Check sheet for the modelled part. Datum: model origin and axes. Units: mm. A direction names the side the tool comes from. Give positions to 0.01 mm unless a question says otherwise; leave off trailing zeros. Write each loop counter-clockwise with the first axis right and the second up, starting at its lowest first coordinate (ties: lowest second). Pieces come first, ordered by that corner, then holes. Notation, with made-up numbers: (59.5, -4.5) -> (81.5, -4.5) arc R28 ccw to (81.5, 16.5) -> close; hole circle Ø4 at (85.25, 19). An arc over 180 degrees is marked (long way). Use a Markdown table: item, result. Add a question column.
1. Gauge pin test, flat ends, axial feed: P1, Ø10, axis at y = 31, z = 32, coming from the -X side; P2, Ø16.5, axis at x = 36, y = 30.5, coming from the -Z side; P3, Ø2.5, axis at y = 51.5, z = -15.5, coming from the -X side; P4, Ø1, axis at x = 34.5, z = 134, coming from the +Y side. Record the tip position at first contact, or that the pin passes through.
2. Set-up check for faces 1 (the flat face through (33, 45, 12)), 2 (the cylindrical face through (239.3, 2.85, 3.01)), 3 (the flat face through (148, 15, 98)), 4 (the cylindrical face through (60.7, 59.99, 2.85)), 5 (the flat face through (260, 45, 148)): record each of +Z, -Z, +X, -X, +Y, -Y from which the full face is reachable in a straight line by a thin tool's end or side.
3. Cross-section at A-A (z = 214). Enter the section's corners in (x, y).
4. Cross-section at B-B (x = 57). Enter the section's corners in (y, z), then the cut area to 3 significant figures.
5. Scan lines: probe 1 along X at (y, z) = (30.1, 167.5); probe 2 along Z at (x, y) = (175, 69); probe 3 along Y at (x, z) = (98.5, 108.5). Record each from-to range of solid material in increasing order. Write a range as [from, to].
6. Cross-section at D-D (y = 75). Enter the section's corners in (x, z), then the cut area to 3 significant figures.
7. Cross-section at C-C (z = 176). Enter the section's corners in (x, y).
8. Release check for a two-part mould opening along Z. For faces 6 (the flat face through (260, 45, 188)), 7 (the cylindrical face through (34.53, 45.07, 168.28)), 8 (the flat face through (5, 31, 82.3)), 9 (the flat face through (33, 45, 148)) record: released by +Z, released by -Z, zero draft, split by the parting line, or undercut.
from build123d import *

# Parameters (mm, degrees)
SKETCH1_W                = 300
SKETCH1_H                = 200
BOSS_EXTRUDE1_DEPTH      = 15
SKETCH3_W                = 33
SKETCH3_H                = 40
BOSS_EXTRUDE2_DEPTH      = 33
SKETCH4_R                = 15.1
CUT_EXTRUDE1_DEPTH       = 222
SKETCH5_W                = 300
SKETCH5_H                = 200
BOSS_EXTRUDE3_DEPTH      = 15
SKETCH6_W                = 100
SKETCH6_H                = 15
BOSS_EXTRUDE4_DEPTH      = 40
BOSS_EXTRUDE4_DEPTH_BACK = 240
FILLET1_R                = 10
BOSS_EXTRUDE7_DEPTH      = 34
FILLET2_R                = 10
FILLET3_R                = 10
SKETCH12_R               = 1
CUT_EXTRUDE4_DEPTH       = 1
SKETCH13_R               = 2.5
CUT_EXTRUDE5_DEPTH       = 27
SKETCH14_R               = 2.5
CUT_EXTRUDE6_DEPTH       = 32
SKETCH15_R               = 50
BOSS_EXTRUDE9_DEPTH      = 30
SKETCH16_R               = 1
CUT_EXTRUDE7_DEPTH       = 63


with BuildPart() as part:
    # Sketch1 → Boss-Extrude1 (new body)
    with BuildSketch(Plane(origin=(0, 0, 0), x_dir=(1, 0, 0), z_dir=(0, 1, 0))):
        with Locations((150, -100)):
            Rectangle(SKETCH1_W, SKETCH1_H)
    extrude(amount=BOSS_EXTRUDE1_DEPTH)

    # Sketch3 → Boss-Extrude2 (add)
    with BuildSketch(Plane(origin=(0, 15, 0), x_dir=(1, 0, 0), z_dir=(0, 1, 0))):
        with Locations((263.5, -168)):
            Rectangle(SKETCH3_W, SKETCH3_H)
        with Locations((263.5, -32)):
            Rectangle(SKETCH3_W, SKETCH3_H)
        with Locations((36.5, -32)):
            Rectangle(SKETCH3_W, SKETCH3_H)
        with Locations((36.5, -168)):
            Rectangle(SKETCH3_W, SKETCH3_H)
    extrude(amount=BOSS_EXTRUDE2_DEPTH)

    # Sketch4 → Cut-Extrude1 (cut)
    with BuildSketch(Plane.XY.offset(188)):
        with Locations((36.5, 30.1)):
            Circle(SKETCH4_R)
        with Locations((263.5, 30.1)):
            Circle(SKETCH4_R)
    extrude(amount=-CUT_EXTRUDE1_DEPTH, mode=Mode.SUBTRACT)

    # Sketch5 → Boss-Extrude3 (add)
    with BuildSketch(Plane(origin=(0, 48, 0), x_dir=(1, 0, 0), z_dir=(0, 1, 0))):
        with Locations((150, -100)):
            Rectangle(SKETCH5_W, SKETCH5_H)
    extrude(amount=BOSS_EXTRUDE3_DEPTH)

    # Sketch6 → Boss-Extrude4 (add, two sides)
    with BuildSketch(Plane(origin=(0, 0, 0), x_dir=(-1, 0, 0), z_dir=(0, 0, -1))) as boss_extrude4_sk:
        with Locations((-150, 55.5)):
            Rectangle(SKETCH6_W, SKETCH6_H)
        with Locations((-150, 7.5)):
            Rectangle(SKETCH6_W, SKETCH6_H)
    extrude(amount=BOSS_EXTRUDE4_DEPTH)
    extrude(boss_extrude4_sk.sketch, amount=-BOSS_EXTRUDE4_DEPTH_BACK)

    # Fillet1
    fillet1_edges = [part.edges().sort_by_distance(p)[0] for p in [
        (100, 55.5, 240),
        (200, 55.5, 240),
        (100, 55.5, -40),
        (200, 55.5, -40),
        (200, 7.5, 240),
        (100, 7.5, 240),
        (200, 7.5, -40),
        (100, 7.5, -40),
        (0, 7.5, 0),
        (300, 7.5, 0),
        (300, 7.5, 200),
        (0, 7.5, 200),
        (0, 55.5, 0),
        (0, 55.5, 200),
        (300, 55.5, 200),
        (300, 55.5, 0),
    ]]
    fillet(fillet1_edges, radius=FILLET1_R)

    # Sketch11 → Boss-Extrude7 (add)
    with BuildSketch(Plane(origin=(0, 15, 0), x_dir=(1, 0, 0), z_dir=(0, 1, 0))):
        Polygon((0, -82.3), (0, -100), (0, -117.7), (10, -117.7), (10, -82.3), align=None)
    extrude(amount=BOSS_EXTRUDE7_DEPTH)

    # Fillet2
    fillet2_edges = [part.edges().sort_by_distance(p)[0] for p in [
        (245, 63, 200),
        (55, 63, 0),
        (200, 63, -15),
        (100, 63, -15),
        (245, 63, 0),
        (300, 63, 100),
        (150, 63, -40),
        (0, 63, 100),
        (55, 63, 200),
        (100, 63, 215),
        (150, 63, 240),
        (200, 63, 215),
        (102.928932188, 63, -37.071067812),
        (197.071067812, 63, -37.071067812),
        (102.928932188, 63, 237.071067812),
        (197.071067812, 63, 237.071067812),
        (297.071067812, 63, 197.071067812),
        (2.928932188, 63, 197.071067812),
        (2.928932188, 63, 2.928932188),
        (297.071067812, 63, 2.928932188),
    ]]
    fillet(fillet2_edges, radius=FILLET2_R)

    # Fillet3
    fillet3_edges = [part.edges().sort_by_distance(p)[0] for p in [
        (55, 0, 0),
        (245, 0, 200),
        (100, 0, -15),
        (200, 0, -15),
        (245, 0, 0),
        (150, 0, -40),
        (300, 0, 100),
        (200, 0, 215),
        (150, 0, 240),
        (100, 0, 215),
        (55, 0, 200),
        (0, 0, 100),
        (197.071067812, 0, -37.071067812),
        (102.928932188, 0, -37.071067812),
        (102.928932188, 0, 237.071067812),
        (197.071067812, 0, 237.071067812),
        (297.071067812, 0, 197.071067812),
        (2.928932188, 0, 197.071067812),
        (2.928932188, 0, 2.928932188),
        (297.071067812, 0, 2.928932188),
    ]]
    fillet(fillet3_edges, radius=FILLET3_R)

    # Sketch12 → Cut-Extrude4 (cut)
    with BuildSketch(Plane.ZY):
        with Locations((100, 31.5)):
            Circle(SKETCH12_R)
    extrude(amount=-CUT_EXTRUDE4_DEPTH, mode=Mode.SUBTRACT)

    # Sketch13 → Cut-Extrude5 (cut)
    with BuildSketch(Plane(origin=(0, 63, 0), x_dir=(1, 0, 0), z_dir=(0, 1, 0))):
        with Locations((150, -100)):
            Circle(SKETCH13_R)
    extrude(amount=-CUT_EXTRUDE5_DEPTH, mode=Mode.SUBTRACT)

    # Sketch14 → Cut-Extrude6 (cut)
    with BuildSketch(Plane(origin=(0, 63, 0), x_dir=(1, 0, 0), z_dir=(0, 1, 0))):
        with Locations((20, -131)):
            Circle(SKETCH14_R)
        with Locations((20, -69)):
            Circle(SKETCH14_R)
        with Locations((77, -75)):
            Circle(SKETCH14_R)
        with Locations((77, -125)):
            Circle(SKETCH14_R)
    extrude(amount=-CUT_EXTRUDE6_DEPTH, mode=Mode.SUBTRACT)

    # Sketch15 → Boss-Extrude9 (add)
    with BuildSketch(Plane(origin=(0, 63, 0), x_dir=(1, 0, 0), z_dir=(0, 1, 0))):
        with Locations((175, -100)):
            Circle(SKETCH15_R)
    extrude(amount=BOSS_EXTRUDE9_DEPTH)

    # Sketch16 → Cut-Extrude7 (cut)
    with BuildSketch(Plane(origin=(0, 93, 0), x_dir=(1, 0, 0), z_dir=(0, 1, 0))):
        with Locations((175, -100)):
            Circle(SKETCH16_R)
    extrude(amount=-CUT_EXTRUDE7_DEPTH, mode=Mode.SUBTRACT)


solid = part.part
Worked answers:
| question | item | result |
|---|---|---|
| 1 | P1 | stops at x = 20 |
| 1 | P2 | passes through |
| 1 | P3 | stops at x = 100 |
| 1 | P4 | stops at y = 63 |
| 2 | face 1 | -Z, +X, -X |
| 2 | face 2 | -Z, +X, -Y |
| 2 | face 3 | none |
| 2 | face 4 | -Z, -X, +Y |
| 2 | face 5 | +X, -X |
| 3 | outline | (100, 10) arc R10 ccw to (110, 0) -> (190, 0) arc R10 ccw to (200, 10) -> (200, 15) -> (100, 15) -> close; (100, 48) -> (200, 48) -> (200, 53) arc R10 ccw to (190, 63) -> (110, 63) arc R10 ccw to (100, 53) -> close |
| 4 | outline | (0, 10) arc R10 ccw to (10, 0) -> (15, 0) -> (15, 200) -> (10, 200) arc R10 ccw to (0, 190) -> close; (48, 0) -> (53, 0) arc R10 ccw to (63, 10) -> (63, 190) arc R10 ccw to (53, 200) -> (48, 200) -> close |
| 4 | area | 5,910 mm² |
| 5 | probe 1 | x = [20, 21.4], [51.6, 53], [247, 248.4], [278.6, 280] |
| 5 | probe 2 | z = [50, 99], [101, 150] |
| 5 | probe 3 | y = [0, 15], [48, 63] |
| 6 | outline | circle Ø100 at (175, 100); hole circle Ø2 at (175, 100) |
| 6 | area | 7,850 mm² |
| 7 | outline | (0, 10) arc R10 ccw to (10, 0) -> (290, 0) arc R10 ccw to (300, 10) -> (300, 15) -> (280, 15) -> (280, 48) -> (300, 48) -> (300, 53) arc R10 ccw to (290, 63) -> (10, 63) arc R10 ccw to (0, 53) -> (0, 48) -> (20, 48) -> (20, 15) -> (0, 15) -> close; hole circle Ø30.2 at (36.5, 30.1); hole (53, 15) -> (247, 15) -> (247, 48) -> (53, 48) -> close; hole circle Ø30.2 at (263.5, 30.1) |
| 8 | face 6 | released by +Z |
| 8 | face 7 | zero draft |
| 8 | face 8 | released by -Z |
| 8 | face 9 | undercut |
